Model file for the job. Use its own axes, mm. Round coordinates to 2 decimals unless told otherwise and drop trailing zeros. Loops run counter-clockwise (first coordinate to the right, second up) from the corner with the lowest first, then second, coordinate; pieces in that order, holes last. Notation, with made-up numbers: (76.25, -21) - (126.25, -21) arc R25 ccw to (126.25, -5) - close; hole circle Ø11 at (8, 43). An arc over 180 degrees is marked (long way). Use one line per item in the form item = value.
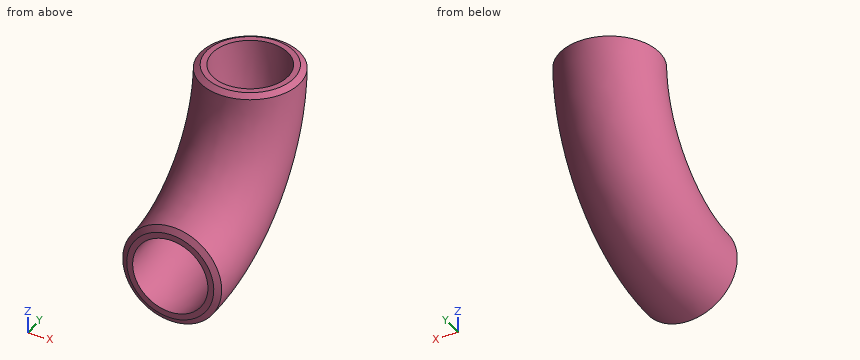
from build123d import *

# Parameters (mm, degrees)
ROHR_R   = 13.45
ROHR_R_2 = 10.25


with BuildPart() as part:
    # Bogen: sweep along a path in Pfad
    with BuildLine(Plane(origin=(0, 0, 0), x_dir=(0, 0, -1), z_dir=(1, 0, 0))) as bogen_path:
        ThreePointArc((0, -38), (-11.129942315, -11.129942315), (-38, 0))
    # Rohr → Bogen (sweep)
    with BuildSketch(Plane(origin=(0, -38, 0), x_dir=(-1, 0, 0), z_dir=(0, -1, 0))):
        Circle(ROHR_R)
        Circle(ROHR_R_2, mode=Mode.SUBTRACT)
    sweep(path=bogen_path.line)

    # SkzFase one side → Fase1 (revolve, cut)
    with BuildSketch(Plane(origin=(0, 0, 0), x_dir=(0, 0, -1), z_dir=(1, 0, 0)), mode=Mode.PRIVATE) as fase1_sk:
        Polygon((15.45, -35.921539031), (11.85, -38), (15.45, -38), align=None)
    revolve(fase1_sk.sketch.rotate(Axis((0, 0, 0), (0, -1, 0)), 180), axis=Axis((0, 0, 0), (0, -1, 0)), mode=Mode.SUBTRACT)  # turned: the seam where the file's is

    # Skizze1_3 → Fase2 (revolve, cut)
    with BuildSketch(Plane(origin=(0, 0, 0), x_dir=(0, 0, -1), z_dir=(1, 0, 0))):
        Polygon((-35.921539031, 15.45), (-38, 11.85), (-38, 15.45), align=None)
    revolve(axis=Axis((0, 0, 0), (0, 0, 1)), mode=Mode.SUBTRACT)


solid = part.part
1. Flat gauge pins, fed straight in: pin 1 (1.5 mm diameter, centred on x = 0, z = 31, fed in from +Y); pin 2 (1 mm diameter, centred on y = -23, z = 14, fed in from -X); pin 3 (8 mm diameter, centred on y = -16.5, z = 14, fed in from -X); pin 4 (1 mm diameter, centred on y = -19.5, z = 25.5, fed in from +X). Where does each tip first touch, or does it go through?
Geometry check:
pin_1 = 13.07
pin_2 = -9.81
pin_3 = -13.33
pin_4 = through
2. Wall check: probe 1 along X at (y, z) = (-29.5, -0.5); probe 2 along Y at (x, z) = (-8.5, 14); probe 3 along X at (y, z) = (-21.5, 9.5). Give the ranges that are in metal, low to high.
Geometry check:
probe_1 = -13.37 to -10.15, 10.15 to 13.37
probe_2 = -24.42 to -16.43, -1.45 to 4.06
probe_3 = -12.46 to -8.91, 8.91 to 12.46
3. Cut at A-A, the plane x = 0. Give the cut face in (y, z), plus the area to 3 significant figures.
Geometry check:
outline = (-38, -11.85) - (-37.08, -13.44) arc R51.45 ccw to (13.44, 37.08) - (11.85, 38) - (10.25, 38) arc R48.25 cw to (-38, -10.25) - close; (-38, 10.25) arc R27.75 ccw to (-10.25, 38) - (-11.85, 38) - (-13.47, 37.07) arc R24.55 cw to (-37.07, 13.47) - (-38, 11.85) - close
area = 379 mm^2
